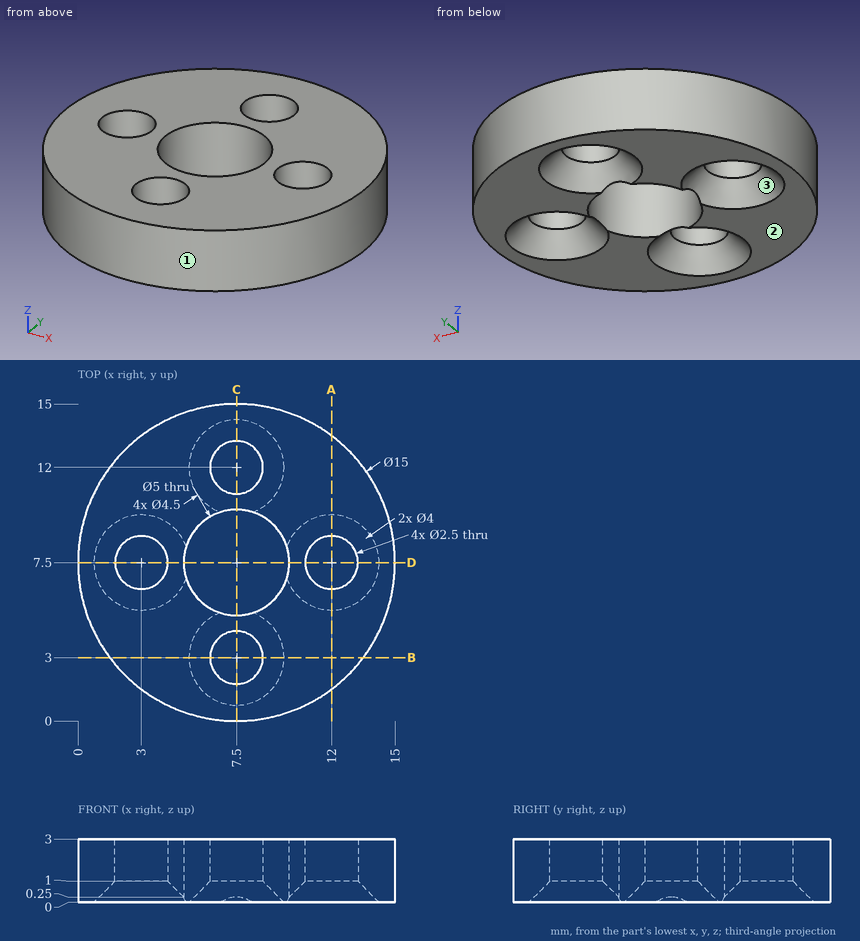
Check sheet for the drawn part. Datum: minimum x, y, z corner. Units: mm. Round coordinates to 2 decimals unless told otherwise and drop trailing zeros. Order: outer loops, then holes, each group sorted by start corner. A loop starts at its lowest first (then second) coordinate and runs counter-clockwise, first axis right, second up. Notation, with made-up numbers: (-25, 86) -> (-17, 86) arc R23 cw to (-17, 124) -> close; hole circle Ø10 at (0.5, -34). An arc over 180 degrees is marked (long way). Put each result on its own line as item: value.
1) Material ranges on line 1 (Y direction, x = 7.5, z = 2); line 2 (X direction, y = 8.75, z = 0.7); line 3 (X direction, y = 7, z = 0.95), recorded low to high.
Final values:
line 1: y = 0 to 1.75, 4.25 to 5, 10 to 10.75, 13.25 to 15
line 2: x = 0.1 to 2.08, 3.92 to 5.33, 9.67 to 11.08, 12.92 to 14.9
line 3: x = 0.02 to 1.8, 4.2 to 5.05, 9.95 to 10.8, 13.2 to 14.98
2) Depth check by flat-ended pin: pin 1 (1.5 mm diameter, centred on y = 2.5, z = 1, fed in from +X); pin 2 (1.5 mm diameter, centred on y = 9.5, z = 2.5, fed in from -X); pin 3 (4 mm diameter, centred on x = 7.5, y = 3, fed in from -Z); pin 4 (1.5 mm diameter, centred on x = 7.5, y = 12, fed in from +Z). Enter the tip coordinate at first touch or a pass-through.
Final values:
pin 1: stops at x = 13.68
pin 2: stops at x = 0.1
pin 3: stops at z = 0.25
pin 4: passes through
3) Section check C-C (x = 7.5). Record the cut outline in (y, z), then the cut area to 3 significant figures.
Final values:
outline: (0, 0) -> (0.75, 0) -> (1.75, 1) -> (1.75, 3) -> (0, 3) -> close; (4.25, 1) -> (5, 0.25) -> (5, 3) -> (4.25, 3) -> close; (10, 0.25) -> (10.75, 1) -> (10.75, 3) -> (10, 3) -> close; (13.25, 1) -> (14.25, 0) -> (15, 0) -> (15, 3) -> (13.25, 3) -> close
area: 13.1 mm^2
4) Section check A-A (x = 12). Record the cut outline in (y, z), then the cut area to 3 significant figures.
Final values:
outline: (1.5, 0) -> (5.25, 0) -> (6.25, 1) -> (6.25, 3) -> (1.5, 3) -> close; (8.75, 1) -> (9.75, 0) -> (13.5, 0) -> (13.5, 3) -> (8.75, 3) -> close
area: 27.5 mm^2
5) Mould release check, pull along X, two halves, no side actions. Record for the marked faces 1, 2 and 3: +X half, -X half, draft (parallel to the pull), parting line (faces both ways), or undercut.
Final values:
face 1: parting line
face 2: draft
face 3: undercut
